Autodesk Inventor part; units mm, degrees
ref_plane "YZ Plane" through (0, 0, 0) normal (1, 0, 0) x (0, 1, 0)
ref_plane "XZ Plane" through (0, 0, 0) normal (0, 1, 0) x (-1, 0, 0)
ref_plane "XY Plane" through (0, 0, 0) normal (0, 0, 1) x (1, 0, 0)
sketch "Sketch1" plane through (0, 0, 0) normal (0, 1, 0) x (-1, 0, 0)
  line L0 (0, 0) -> (0, 5)
  line L1 (0, 5) -> (7, 5)
  line L2 (7, 5) -> (7, -15)
  line L3 (7, -15) -> (0, -15)
  line L4 (0, -15) -> (0, -10)
  line L5 (0, -10) -> (4, -10)
  line L6 (4, -10) -> (4, 0)
  line L7 (4, 0) -> (0, 0)
  dimension "d0" = 5
  dimension "d1" = 7
  dimension "d2" = 20
  dimension "d3" = 7
  dimension "d4" = 5
  dimension "d5" = 4
  dimension "d6" = 10
extrude "Extrusion1" add sketch "Sketch1" along normal blind 40
sketch "Sketch2" plane through (-7, 0, -15) normal (-1, 0, 0) x (0, 0, 1)
  line L0 (5, 0) -> (5, 40)
  line L1 (15, 0) -> (15, 40)
  point P0 (15, 20)
  point P1 (10, 10)
  point P2 (10, 30)
  dimension "d9" = 5
  dimension "d10" = 10
  dimension "d11" = 20
  dimension "d12" = 10
sketch "Sketch5" plane through (0, 0, 0) normal (0, -1, 0) x (1, 0, 0)
  line L0 (-1, -10) -> (-1, -9.5)
  line L1 (-1.5, -9) -> (-1.5, -9)
  line L2 (-2, -9.5) -> (-2, -10)
  line L3 (-2, -10) -> (-1, -10)
  line L4 (-1, -0.5) -> (-1, 0)
  line L5 (-1, 0) -> (-2, 0)
  line L6 (-2, 0) -> (-2, -0.5)
  line L7 (-1.5, -1) -> (-1.5, -1)
  arc A0 (-1.5, -9) -> (-2, -9.5) centre (-1.5, -9.5) ccw
  arc A1 (-1, -9.5) -> (-1.5, -9) centre (-1.5, -9.5) ccw
  arc A2 (-2, -0.5) -> (-1.5, -1) centre (-1.5, -0.5) ccw
  arc A3 (-1.5, -1) -> (-1, -0.5) centre (-1.5, -0.5) ccw
  point P0 (0, 0)
  point P1 (-1, -9)
  point P2 (-2, -9)
  point P3 (-1, -1)
  point P4 (-2, -1)
  point P5 (-1.5, 0)
  point P6 (-1.5, -10)
  point P7 (0, -10)
  dimension "d35" = 1
  dimension "d36" = 1
  dimension "d37" = 1
  dimension "d38" = 1
  dimension "d39" = 1
  dimension "d40" = 1
  dimension "d41" = 0.5
  dimension "d42" = 1
  dimension "d43" = 1
extrude "Extrusion2" add sketch "Sketch5" against normal blind 40
sketch "Sketch10" plane through (-7, 0, -15) normal (-1, 0, 0) x (0, 0, 1)
  circle A0 centre (2.5, 12) radius 1.5
  circle A1 centre (2.5, 28) radius 1.5
  circle A2 centre (17.5, 12) radius 1.5
  circle A3 centre (17.5, 28) radius 1.5
  line L0 (20, 0) -> (0, 0)
  line L1 (0, 0) -> (0, 40)
  point P0 (15, 0)
  dimension "d72" = 3
  dimension "d73" = 3
  dimension "d74" = 3
  dimension "d75" = 3
  dimension "d76" = 16
  dimension "d77" = 15
  dimension "d78" = 15
  dimension "d79" = 16
  dimension "d81" = 2.5
  dimension "d82" = 12
extrude "Extrusion6" cut sketch "Sketch10" against normal blind 3
sketch "Sketch4" plane through (-4, 0, 0) normal (1, 0, 0) x (0, 0, -1)
  point P0 (5, 30)
  point P1 (5, 10)
properties part number "Karetka"
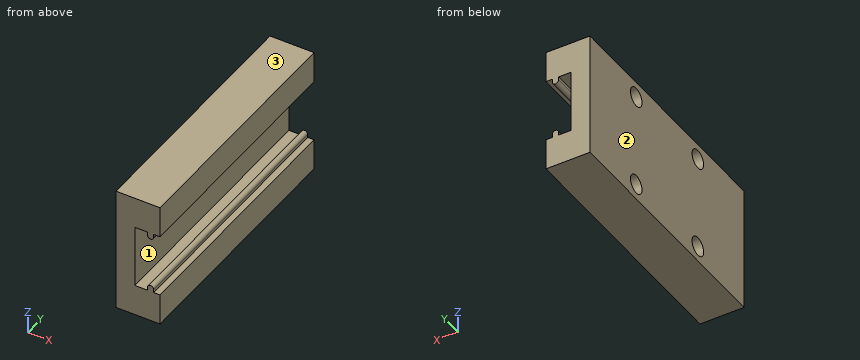
Build history of the part. All positions in model axes, mm. Face numbers are marked on the shaded views. Coordinates: 2 decimals unless noted, no trailing zeros. Write each loop counter-clockwise with the first axis right and the second up, starting at its lowest first coordinate (ties: lowest second). Pieces come first, ordered by that corner, then holes. Notation, with made-up numbers: (-38.75, -1) -> (17.25, -1) arc R31 cw to (17.25, 35) -> close; hole circle Ø11 at (23.25, -14). An arc over 180 degrees is marked (long way). Use CSV: the item, a comma, the result in double quotes. Start each with the question number.
Q1. Cut at A-A, the plane x = -3.5. List the corners of the cut face in (y, z).
Q2. Cut at D-D, the plane x = -6.25. List the corners of the cut face in (y, z).
Q3. Cut at C-C, the plane y = 18.5. List the corners of the cut face in (x, z), then the cut area to 3 significant figures.
Q4. Pull direction Z, two halves, no side cores. Call the marked faces 1, 2 and 3: released by +Z, released by -Z, zero draft, split by the parting line, or undercut.
Q5. Flat gauge pins, fed straight in: pin 1 Ø1.5 at (y, z) = (12.5, -13) entering from -X; pin 2 Ø8 at (y, z) = (26, -5.5) entering from +X. Where does each tip first touch, or does it go through?
Q6. Drill centre lines: probe 1 along Y at (x, z) = (-6.3, -12.5); probe 2 along Z at (x, y) = (-2.25, 35); probe 3 along Z at (x, y) = (-1.5, 11.5). Where is each one in solid material? Low to high.
Q7. Cut at B-B, the plane z = -12.5. List the corners of the cut face in (x, y), then the cut area to 3 significant figures.
Checked values:
1,outline,"(0, -15) -> (40, -15) -> (40, -10) -> (0, -10) -> close; (0, 0) -> (40, 0) -> (40, 5) -> (0, 5) -> close"
2,outline,"(0, -15) -> (40, -15) -> (40, 5) -> (0, 5) -> close; hole circle Ø3 at (12, -12.5); hole circle Ø3 at (12, 2.5); hole circle Ø3 at (28, -12.5); hole circle Ø3 at (28, 2.5)"
3,outline,"(-7, -15) -> (0, -15) -> (0, -10) -> (-1, -10) -> (-1, -9.5) arc R0.5 ccw to (-2, -9.5) -> (-2, -10) -> (-4, -10) -> (-4, 0) -> (-2, 0) -> (-2, -0.5) arc R0.5 ccw to (-1, -0.5) -> (-1, 0) -> (0, 0) -> (0, 5) -> (-7, 5) -> close"
3,area,"102 mm²"
4,face 1,"undercut"
4,face 2,"zero draft"
4,face 3,"released by +Z"
5,pin 1,"stops at x = -4"
5,pin 2,"stops at x = -1"
6,probe 1,"y = 0 to 10.5, 13.5 to 26.5, 29.5 to 40"
6,probe 2,"z = -15 to -10, 0 to 5"
6,probe 3,"z = -15 to -9, -1 to 5"
7,outline,"(-7, 0) -> (0, 0) -> (0, 40) -> (-7, 40) -> (-7, 29.5) -> (-4, 29.5) -> (-4, 26.5) -> (-7, 26.5) -> (-7, 13.5) -> (-4, 13.5) -> (-4, 10.5) -> (-7, 10.5) -> close"
7,area,"262 mm²"
